Geometry: final body of the model. Coordinates: model frame, mm. A direction names the side the tool comes from. Coordinates: 2 decimals unless noted, no trailing zeros. Order: outer loops, then holes, each group sorted by start corner. A loop starts at its lowest first (then second) coordinate and runs counter-clockwise, first axis right, second up. Notation, with made-up numbers: M -10,75 L 30,75 A19 ccw 30,106 Z; hole C -16,-30.75 d9. An arc over 180 degrees is marked long. Write item = value, one per line.
Autodesk Fusion 360 part; units mm, degrees
sketch "Skizze1" plane through (0, 0, 0) normal (0, 0, 1) x (1, 0, 0)
  line L0 (0, 0) -> (100, 0)
  line L1 (100, 0) -> (100, 10)
  line L2 (100, 10) -> (0, 10)
  line L3 (0, 10) -> (0, 0)
sketch "Skizze2" plane through (0, 0, 0) normal (1, 0, 0) x (0, 1, 0)
  line L0 (10, 0) -> (0, 0)
  line L1 (2, 14) -> (2, 0)
  line L2 (9, 0) -> (9, 14)
  line L3 (2, 14) -> (3, 14)
  line L4 (3, 14) -> (0, 16)
  line L5 (0, 16) -> (0, 0)
  line L6 (9, 14) -> (8, 14)
  line L7 (8, 14) -> (11, 16)
  line L8 (11, 16) -> (11, 0)
  line L9 (11, 0) -> (11, -2)
  line L10 (11, -2) -> (0, -2)
  line L11 (0, -2) -> (0, 0)
  line L12 (0, 16) -> (-0.5, -2)
  line L13 (-0.5, -2) -> (0, -2)
  line L14 (11, 16) -> (11.5, -2)
  line L15 (11, -2) -> (11.5, -2)
  dimension "d1" = 7
  dimension "d3" = 5
  dimension "d4" = 14
  dimension "d6" = 2
  dimension "d7" = 2
  dimension "d9" = 2
  dimension "d10" = 2
  dimension "d11" = 11
  dimension "d13" = 2
  dimension "d18" = 12
extrude "Extrusion1" add sketch "Skizze2" along normal blind 60
fillet "Abrundung1" radius 0.2 10 faces at (20, 8.6667, 14) (20, 9, 14.6667) (20, 2.3333, 14) (20, 2, 9.3333) (20, 2, 14.6667) (60, 1.1667, 4) (20, 3.5, -2) (0, 1.1667, 4) (20, 9, 4.6667) (20, 6.6667, 0)
1) Mould query, pull axis Y, two halves, no side actions, for faces 4 (the face through (30, 6, 0)), 5 (the face through (29.583, 1.391, 15.073)), 6 (the face through (0, 1.6, 5.1)). Classes: pulls with the +Y half, pulls with the -Y half, needs draft (parallel to the pull), parting line crosses it, or undercut.
Numbers:
face_4 = undercut
face_5 = undercut
face_6 = needs draft
2) Set-up query: faces 1 (the face through (59.94, 9.671, 15.046)), 2 (the face through (30, 2, 7)), 3 (the face through (29.583, 9.609, 15.073)). Return all of +Z, -Z, +X, -X, +Y, -Y with unobstructed straight access to the full face (end or side cutting, diameter ignored); none if empty.
Numbers:
face_1 = +Z, +X
face_2 = +X, -X
face_3 = +Z, +X, -X
3) Section B-B, the plane y = 4.75. Return loops of the section in (x, z).
Numbers:
outline = M 0,-1.8 A0.2 ccw 0.2,-2 L 59.8,-2 A0.2 ccw 60,-1.8 L 60,-0.2 A0.2 ccw 59.8,0 L 0.2,0 A0.2 ccw 0,-0.2 Z
4) Section A-A, the plane x = 20. Return loops of the section in (y, z), and give its area (3 significant figures).
Numbers:
outline = M -0.49,-1.79 A0.2 ccw -0.29,-2 L 11.29,-2 A0.2 ccw 11.49,-1.79 L 11.01,15.64 A0.2 ccw 10.7,15.8 L 8.55,14.37 A0.2 ccw 8.66,14 L 8.8,14 A0.2 cw 9,13.8 L 9,0.2 A0.2 cw 8.8,0 L 2.2,0 A0.2 cw 2,0.2 L 2,13.8 A0.2 cw 2.2,14 L 2.34,14 A0.2 ccw 2.45,14.37 L 0.3,15.8 A0.2 ccw -0.01,15.64 Z
area = 92.8 mm²
5) Pin query (flat end, axial travel): pin 1 (2 mm diameter, centred on x = 11.5, z = 6.5, fed in from +Y); pin 2 (5.5 mm diameter, centred on x = 19.5, y = 5.5, fed in from +Z); pin 3 (1 mm diameter, centred on x = 48, z = 11.5, fed in from +Y). Return the tip coordinate at first contact, or that it passes through.
Numbers:
pin_1 = 11.29
pin_2 = 0
pin_3 = 11.14
6) Line query: L1, parallel to Z at x = 33.5, y = 7; L2, parallel to Y at x = 32, z = 12.75; L3, parallel to Y at x = 4, z = 14.25. Output: solid intervals per line, ascending.
Numbers:
L1 = -2 to 0
L2 = -0.09 to 2, 9 to 11.09
L3 = -0.05 to 2.53, 8.47 to 11.05
